Input: part model. Units: mm. Frame: model coordinates. A direction names the side the tool comes from. Give positions to 0.01 mm unless a question says otherwise; leave off trailing zeros. Loops run counter-clockwise (first coordinate to the right, second up) from the corner with the lowest first, then second, coordinate; pieces in that order, holes last. Notation, with made-up numbers: (40, 40) - (90, 40) arc R20 ccw to (90, 75) - close; hole circle Ø1 at (25.5, 21.5). An arc over 180 degrees is marked (long way). One line per item, written item: value.
from build123d import *

# Parameters (mm, degrees)
SKETCH_R     = 12
SKETCH_W     = 60
SKETCH_H     = 60
PAD_DEPTH    = 30
PAD001_DEPTH = 30


with BuildPart() as part:
    # Sketch → Pad (new body)
    with BuildSketch(Plane.XY):
        with BuildLine():
            Line((-59.342312, -134.143673), (59.515305, -134.143673))
            ThreePointArc((59.515305, -134.143673), (74.047401, -128.124281), (80.066793, -113.592185))
            Line((80.066793, -113.592185), (80.066793, 100.872214))
            ThreePointArc((80.066793, 100.872214), (74.213582, 115.003116), (60.08268, 120.856327))
            Line((60.08268, 120.856327), (-59.689381, 120.856327))
            ThreePointArc((-59.689381, 120.856327), (-74.003928, 114.927048), (-79.933207, 100.612501))
            Line((-79.933207, 100.612501), (-79.933207, -113.552778))
            ThreePointArc((-79.933207, -113.552778), (-73.902274, -128.112739), (-59.342312, -134.143673))
        make_face()
        with Locations((0.120778, 29.919195)):
            Circle(SKETCH_R, mode=Mode.SUBTRACT)
        with Locations((-53.325886, -24.171413)):
            Circle(SKETCH_R, mode=Mode.SUBTRACT)
        with Locations((55.271923, 86.295181)):
            Circle(SKETCH_R, mode=Mode.SUBTRACT)
        with Locations((-0.129082, -90.192567)):
            Rectangle(SKETCH_W, SKETCH_H, mode=Mode.SUBTRACT)
    extrude(amount=PAD_DEPTH)

    # Sketch → Pad001 (join)
    with BuildSketch(Plane.XY):
        with BuildLine():
            Line((-59.342312, -134.143673), (59.515305, -134.143673))
            ThreePointArc((59.515305, -134.143673), (74.047401, -128.124281), (80.066793, -113.592185))
            Line((80.066793, -113.592185), (80.066793, 100.872214))
            ThreePointArc((80.066793, 100.872214), (74.213582, 115.003116), (60.08268, 120.856327))
            Line((60.08268, 120.856327), (-59.689381, 120.856327))
            ThreePointArc((-59.689381, 120.856327), (-74.003928, 114.927048), (-79.933207, 100.612501))
            Line((-79.933207, 100.612501), (-79.933207, -113.552778))
            ThreePointArc((-79.933207, -113.552778), (-73.902274, -128.112739), (-59.342312, -134.143673))
        make_face()
        with Locations((0.120778, 29.919195)):
            Circle(SKETCH_R, mode=Mode.SUBTRACT)
        with Locations((-53.325886, -24.171413)):
            Circle(SKETCH_R, mode=Mode.SUBTRACT)
        with Locations((55.271923, 86.295181)):
            Circle(SKETCH_R, mode=Mode.SUBTRACT)
        with Locations((-0.129082, -90.192567)):
            Rectangle(SKETCH_W, SKETCH_H, mode=Mode.SUBTRACT)
    extrude(amount=PAD001_DEPTH)


solid = part.part
Item 1: Section C-C, the plane z = 7. Output: boundary loops of the cut face in (x, y), and give its area (3 significant figures).
Verdict:
outline: (-79.93, -113.55) arc R20.59 ccw to (-59.34, -134.14) - (59.52, -134.14) arc R20.55 ccw to (80.07, -113.59) - (80.07, 100.87) arc R19.98 ccw to (60.08, 120.86) - (-59.69, 120.86) arc R20.24 ccw to (-79.93, 100.61) - close; hole circle Ø24 at (-53.33, -24.17); hole (-30.13, -120.19) - (29.87, -120.19) - (29.87, -60.19) - (-30.13, -60.19) - close; hole circle Ø24 at (0.12, 29.92); hole circle Ø24 at (55.27, 86.3)
area: 35,500 mm^2
Item 2: Draft query along Y for faces 1 (the face through (1, 120.856, 15)), 2 (the face through (-1, -120.193, 15)), 3 (the face through (80.067, -8, 15)). Return one class per face: pulls with the +Y half, pulls with the -Y half, needs draft (parallel to the pull), parting line crosses it, or undercut.
Verdict:
face 1: pulls with the +Y half
face 2: undercut
face 3: needs draft
Item 3: Section A-A, the plane y = -77.5. Output: boundary loops of the cut face in (x, z), and give its area (3 significant figures).
Verdict:
outline: (-79.93, 0) - (-30.13, 0) - (-30.13, 30) - (-79.93, 30) - close; (29.87, 0) - (80.07, 0) - (80.07, 30) - (29.87, 30) - close
area: 3,000 mm^2
Item 4: Pin query (flat end, axial travel): P1, Ø1.5, axis at x = -36.5, y = -75.5, coming from the -Z side. Return the tip coordinate at first contact, or that it passes through.
Verdict:
P1: stops at z = 0
Item 5: Material intervals for L1, parallel to X at y = -114, z = 9.75; L2, parallel to Y at x = 27.5, z = 18.75; L3, parallel to Y at x = -3.5, z = 14.25, sorted ascending.
Verdict:
L1: x = -79.93 to -30.13, 29.87 to 80.06
L2: y = -134.14 to -120.19, -60.19 to 120.86
L3: y = -134.14 to -120.19, -60.19 to 18.48, 41.36 to 120.86
Item 6: Access query for faces 4 (the face through (-79.933, -5, 15)), 5 (the face through (-30.129, -91, 15)). Directions: +Z, -Z, +X, -X, +Y, -Y. A direction counts if a zero-diameter tool reaches every point of the face in a straight line with its end or side. Return the directions, or none.
Verdict:
face 4: +Z, -Z, -X, +Y, -Y
face 5: +Z, -Z
Item 7: Section B-B, the plane x = -20. Output: boundary loops of the cut face in (y, z).
Verdict:
outline: (-134.14, 0) - (-120.19, 0) - (-120.19, 30) - (-134.14, 30) - close; (-60.19, 0) - (120.86, 0) - (120.86, 30) - (-60.19, 30) - close
